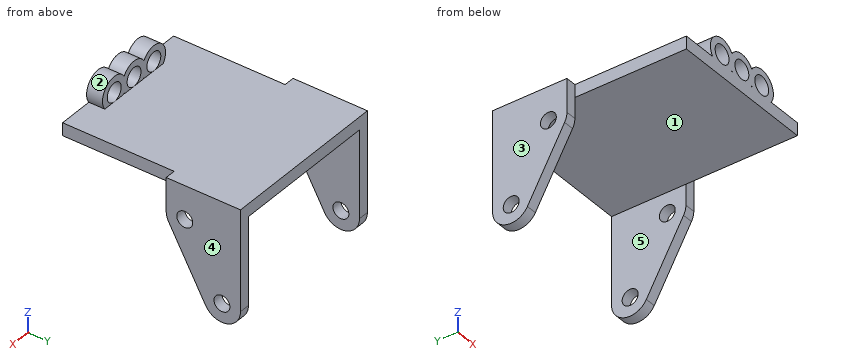
```python
from build123d import *

# Parameters (mm, degrees)
SKETCH2_R                = 2.95
SKETCH2_R_2              = 1.75
EXTRUDE_THIN1_DEPTH      = 3
EXTRUDE_THIN2_DEPTH      = 14
EXTRUDE_THIN2_DEPTH_BACK = 14
SKETCH3_W                = 2.4
SKETCH3_H                = 35
SKETCH4_R                = 1.5
BOSS_EXTRUDE1_DEPTH      = 2
BOSS_EXTRUDE2_START      = -30
SKETCH4_2_R              = 1.5
BOSS_EXTRUDE2_DEPTH      = 2


with BuildPart() as part:
    # Sketch2 → Extrude-Thin1 (new body)
    # profile 1 of 3: a face of its own
    with BuildSketch(Plane(origin=(0, 0, 0), x_dir=(1, 0, 0), z_dir=(0, 1, 0))):
        Circle(SKETCH2_R)
        Circle(SKETCH2_R_2, mode=Mode.SUBTRACT)
    # profile 2 of 3: a face of its own
    with BuildSketch(Plane(origin=(0, 0, 0), x_dir=(1, 0, 0), z_dir=(0, 1, 0))):
        with Locations((5, 0)):
            Circle(SKETCH2_R)
        with Locations((5, 0)):
            Circle(SKETCH2_R_2, mode=Mode.SUBTRACT)
    # profile 3 of 3: a face of its own
    with BuildSketch(Plane(origin=(0, 0, 0), x_dir=(1, 0, 0), z_dir=(0, 1, 0))):
        with Locations((-5, 0)):
            Circle(SKETCH2_R)
        with Locations((-5, 0)):
            Circle(SKETCH2_R_2, mode=Mode.SUBTRACT)
    extrude(amount=EXTRUDE_THIN1_DEPTH)

    # Sketch3 → Extrude-Thin2 (add, two sides: drawn at the far end of the back side and taken through both)
    with BuildSketch(Plane(origin=(0, 0, 0), x_dir=(0, 0, -1), z_dir=(1, 0, 0)).offset(-EXTRUDE_THIN2_DEPTH_BACK)):
        with Locations((2.95, 17.5)):
            Rectangle(SKETCH3_W, SKETCH3_H)
    extrude(amount=EXTRUDE_THIN2_DEPTH + EXTRUDE_THIN2_DEPTH_BACK)

    # Sketch4 → Boss-Extrude1 (add)
    with BuildSketch(Plane(origin=(14, 0, 0), x_dir=(0, 0, -1), z_dir=(1, 0, 0))):
        with BuildLine():
            Line((20.65, 35), (1.75, 35))
            Line((1.75, 35), (1.75, 21))
            Line((1.75, 21), (8.04152842, 21))
            ThreePointArc((8.04152842, 21), (8.918989705, 21.111776027), (9.740405769, 21.439964746))
            Line((9.740405769, 21.439964746), (22.348877349, 28.439964746))
            ThreePointArc((22.348877349, 28.439964746), (24.038223973, 32.377461285), (20.65, 35))
        make_face()
        with Locations(Location((20.65, 31.5, 0), (0, 0, 90))):
            Circle(SKETCH4_R, mode=Mode.SUBTRACT)
        with Locations(Location((8.04152842, 24.5, 0), (0, 0, 90))):
            Circle(SKETCH4_R, mode=Mode.SUBTRACT)
    extrude(amount=BOSS_EXTRUDE1_DEPTH)

    # Sketch4<2> → Boss-Extrude2 (add)
    with BuildSketch(Plane(origin=(14, 0, 0), x_dir=(0, 0, -1), z_dir=(1, 0, 0)).offset(BOSS_EXTRUDE2_START)):
        with BuildLine():
            Line((20.65, 35), (1.75, 35))
            Line((1.75, 35), (1.75, 21))
            Line((1.75, 21), (8.04152842, 21))
            ThreePointArc((8.04152842, 21), (8.918989705, 21.111776027), (9.740405769, 21.439964746))
            Line((9.740405769, 21.439964746), (22.348877349, 28.439964746))
            ThreePointArc((22.348877349, 28.439964746), (24.038223973, 32.377461285), (20.65, 35))
        make_face()
        with Locations(Location((20.65, 31.5, 0), (0, 0, 90))):
            Circle(SKETCH4_2_R, mode=Mode.SUBTRACT)
        with Locations(Location((8.04152842, 24.5, 0), (0, 0, 90))):
            Circle(SKETCH4_2_R, mode=Mode.SUBTRACT)
    extrude(amount=BOSS_EXTRUDE2_DEPTH)


solid = part.part
```
For this review, take the finished solid that the model builds, in its own axes (mm). Face numbers are marked on the shaded views. A direction names the side the tool comes from. Coordinates: 2 decimals unless noted, no trailing zeros. Order: outer loops, then holes, each group sorted by start corner. A loop starts at its lowest first (then second) coordinate and runs counter-clockwise, first axis right, second up. Notation, with made-up numbers: (31.5, 35) - (47.5, 35) arc R16 ccw to (47.5, 63) - close; hole circle Ø10 at (-34, 14.5). An arc over 180 degrees is marked (long way). Answer as a JSON object with one key per item and string values. Group by question number.
1. For probe 1 along X at (y, z) = (2.4, 0); probe 2 along Z at (x, y) = (5, 1); probe 3 along X at (y, z) = (31.5, -4.5), list the stretches that pass through material, from the lowest coordinate up.
2. We need section D-D on z = -11. State the section outline as (x, y) points, then the cut area to 3 significant figures.
3. We need section C-C on x = -4.5. State the section outline as (y, z) points, then the cut area to 3 significant figures.
4. For the marked faces 4 and 5, list the 3-axis set-ups (+Z, -Z, +X, -X, +Y, -Y) from which the entire face can be reached by the end or side of a thin tool; tool diameter is ignored.
5. Clearance check with flat-ended pins moving along their axes: P1, Ø9.5, axis at x = 3.5, y = 13, coming from the +Z side; P2, Ø1, axis at x = 9, y = 9, coming from the -Z side; P3, Ø2, axis at x = -14.5, z = -3.5, coming from the -Y side; P4, Ø2.5, axis at y = 6, z = -3, coming from the -X side. State where each tip first meets the part, or that it passes through.
6. We need section A-A on y = 31.5. State the section outline as (x, z) points, then the cut area to 3 significant figures.
7. We need section B-B on z = 0. State the section outline as (x, y) points, then the cut area to 3 significant figures.
8. The part is to be moulded in two halves that separate along Z. For the marked faces 1, 2 and 3, say which applies: pulls with the +Z half, pulls with the -Z half, needs draft (parallel to the pull), parting line crosses it, or undercut.
Final values:
{
 "1": {"probe 1": "-7.95 to -6.75, -3.25 to -1.75, 1.75 to 3.25, 6.75 to 7.95", "probe 2": "-4.15 to -1.75, 1.75 to 2.95", "probe 3": "-16 to -14, 14 to 16"},
 "2": {"outline": "(-16, 22.14) - (-14, 22.14) - (-14, 35) - (-16, 35) - close; (14, 22.14) - (16, 22.14) - (16, 35) - (14, 35) - close", "area": "51.4 mm²"},
 "3": {"outline": "(0, -4.15) - (35, -4.15) - (35, -1.75) - (3, -1.75) - (3, -1.68) - (0, -1.68) - close; (0, 1.68) - (3, 1.68) - (3, 2.91) - (0, 2.91) - close", "area": "87.9 mm²"},
 "4": {"face 4": "+Z, -Z, +X, +Y, -Y", "face 5": "-Z, +Y, -Y"},
 "5": {"P1": "z = -1.75", "P2": "z = -4.15", "P3": "y = 0", "P4": "x = -14"},
 "6": {"outline": "(-16, -24.15) - (-14, -24.15) - (-14, -22.15) - (-16, -22.15) - close; (-16, -19.15) - (-14, -19.15) - (-14, -4.15) - (14, -4.15) - (14, -19.15) - (16, -19.15) - (16, -1.75) - (-16, -1.75) - close; (14, -24.15) - (16, -24.15) - (16, -22.15) - (14, -22.15) - close", "area": "145 mm²"},
 "7": {"outline": "(-7.95, 0) - (-6.75, 0) - (-6.75, 3) - (-7.95, 3) - close; (-3.25, 0) - (-1.75, 0) - (-1.75, 3) - (-3.25, 3) - close; (1.75, 0) - (3.25, 0) - (3.25, 3) - (1.75, 3) - close; (6.75, 0) - (7.95, 0) - (7.95, 3) - (6.75, 3) - close", "area": "16.2 mm²"},
 "8": {"face 1": "pulls with the -Z half", "face 2": "undercut", "face 3": "needs draft"}
}
